from build123d import *

# Parameters (mm, degrees)
F0_W     = 100
F0_H     = 50.8
F0_R     = 3
F0_W_2   = 32
F1_DEPTH = 9.525


with BuildPart() as f1:
    # F0 (on Top) → F1 (new body)
    with BuildSketch(Plane.XY):
        with Locations((-16, 0)):
            Rectangle(F0_W, F0_H)
        with BuildLine():
            Line((-59, -13.5), (-39, -13.5))
            ThreePointArc((-39, -13.5), (-36.525126, -14.525126), (-35.5, -17))
            ThreePointArc((-35.5, -17), (-36.525126, -19.474874), (-39, -20.5))
            Line((-39, -20.5), (-59, -20.5))
            ThreePointArc((-59, -20.5), (-62.5, -17), (-59, -13.5))
        make_face(mode=Mode.SUBTRACT)
        with Locations((17, -17)):
            Circle(F0_R, mode=Mode.SUBTRACT)
        with BuildLine():
            ThreePointArc((-59, 13.5), (-62.5, 17), (-59, 20.5))
            Line((-59, 20.5), (-39, 20.5))
            ThreePointArc((-39, 20.5), (-36.525126, 19.474874), (-35.5, 17))
            ThreePointArc((-35.5, 17), (-36.525126, 14.525126), (-39, 13.5))
            Line((-39, 13.5), (-59, 13.5))
        make_face(mode=Mode.SUBTRACT)
        with Locations((17, 17)):
            Circle(F0_R, mode=Mode.SUBTRACT)
        with Locations((50, 0)):
            Rectangle(F0_W_2, F0_H)
        with Locations((51, -17)):
            Circle(F0_R, mode=Mode.SUBTRACT)
        with Locations((51, 17)):
            Circle(F0_R, mode=Mode.SUBTRACT)
    extrude(amount=F1_DEPTH)


solid = f1.part
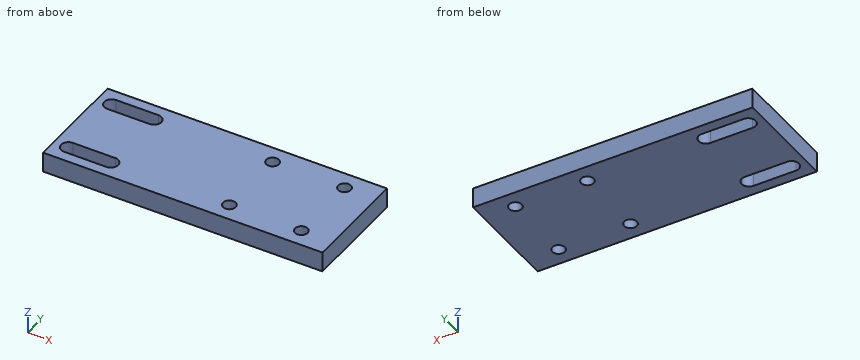
CAD build for the part. Positions are in the model's coordinates, mm. Coordinates: 2 decimals unless noted, no trailing zeros. Order: outer loops, then holes, each group sorted by start corner. A loop starts at its lowest first (then second) coordinate and runs counter-clockwise, first axis right, second up.
Item 1: Band-saw the part on A-A on x = -40.5. List the corners of the cut face in (y, z) (3 decimals).
Check sheet entries:
outline: (-25.4, 0) - (-20.5, 0) - (-20.5, 9.525) - (-25.4, 9.525) - close; (-13.5, 0) - (13.5, 0) - (13.5, 9.525) - (-13.5, 9.525) - close; (20.5, 0) - (25.4, 0) - (25.4, 9.525) - (20.5, 9.525) - close
Item 2: Drill centre lines: L1, parallel to Y at x = -48, z = 7.75; L2, parallel to Y at x = 17, z = 7.25; L3, parallel to X at y = -19, z = 7. Where is each one in solid material? Low to high.
Check sheet entries:
L1: y = -25.4 to -20.5, -13.5 to 13.5, 20.5 to 25.4
L2: y = -25.4 to -20, -14 to 14, 20 to 25.4
L3: x = -66 to -61.87, -36.13 to 14.76, 19.24 to 48.76, 53.24 to 66
Item 3: Band-saw the part on B-B on z = 3.25. List the corners of the cut face in (x, y).
Check sheet entries:
outline: (-66, -25.4) - (66, -25.4) - (66, 25.4) - (-66, 25.4) - close; hole (-59, -20.5) - (-39, -20.5) arc R3.5 ccw to (-35.5, -17) arc R3.5 ccw to (-39, -13.5) - (-59, -13.5) arc R3.5 ccw to start; hole (-59, 13.5) - (-39, 13.5) arc R3.5 ccw to (-35.5, 17) arc R3.5 ccw to (-39, 20.5) - (-59, 20.5) arc R3.5 ccw to start; hole circle Ø6 at (17, -17); hole circle Ø6 at (17, 17); hole circle Ø6 at (51, -17); hole circle Ø6 at (51, 17)
Item 4: Band-saw the part on C-C on x = 17. List the corners of the cut face in (y, z) (3 decimals), plus the area to 3 significant figures.
Check sheet entries:
outline: (-25.4, 0) - (-20, 0) - (-20, 9.525) - (-25.4, 9.525) - close; (-14, 0) - (14, 0) - (14, 9.525) - (-14, 9.525) - close; (20, 0) - (25.4, 0) - (25.4, 9.525) - (20, 9.525) - close
area: 370 mm2
